Input: part model. Units: mm. Frame: model coordinates. Face numbers are marked on the shaded views. A direction names the side the tool comes from. Coordinates: 2 decimals unless noted, no trailing zeros. Order: outer loops, then holes, each group sorted by start corner. A loop starts at its lowest first (then second) coordinate and runs counter-clockwise, first axis right, second up. Notation, with made-up numbers: (57, -10) -> (69, -10) arc R27 ccw to (69, 20) -> close; hole circle Ø7 at (41.25, 23.25). An arc over 180 degrees is marked (long way). Answer as CSV lines item,"result".
from build123d import *

# Parameters (mm, degrees)
SALIENTE_EXTRUIR1_DEPTH = 30
SALIENTE_EXTRUIR2_DEPTH = 90
CORTAR_EXTRUIR1_DEPTH   = 138.564065
MATRIZC1_COUNT          = 6
CROQUIS4_R              = 15.75
CORTAR_EXTRUIR2_DEPTH   = 103.923048
MATRIZC2_COUNT          = 6


with BuildPart() as part:
    # Croquis1 → Saliente-Extruir1 (new body)
    with BuildSketch(Plane(origin=(0, 0, 0), x_dir=(1, 0, 0), z_dir=(0, 1, 0))):
        Polygon((40, 69.282032303), (-40, 69.282032303), (-80, 0), (-40, -69.282032303), (40, -69.282032303), (80, 0), align=None)
    extrude(amount=SALIENTE_EXTRUIR1_DEPTH)

    # Croquis2 → Saliente-Extruir2 (add)
    with BuildSketch(Plane(origin=(0, 0, 0), x_dir=(1, 0, 0), z_dir=(0, 1, 0))):
        Polygon((20, 34.641016151), (-20, 34.641016151), (-40, 0), (-20, -34.641016151), (20, -34.641016151), (40, 0), align=None)
    extrude(amount=SALIENTE_EXTRUIR2_DEPTH)

    # Croquis3 → Cortar-Extruir1 (cut)
    with BuildSketch(Plane(origin=(60, 0, 34.641016151), x_dir=(0.5, 0, -0.866025404), z_dir=(0.866025404, 0, 0.5))):
        with BuildLine():
            Line((-10, 25), (10, 25))
            ThreePointArc((10, 25), (20, 15), (10, 5))
            Line((10, 5), (-10, 5))
            ThreePointArc((-10, 5), (-20, 15), (-10, 25))
        make_face()
    cortar_extruir1 = extrude(amount=-CORTAR_EXTRUIR1_DEPTH, mode=Mode.SUBTRACT)

    # MatrizC1: Cortar-Extruir1 ×6 about axis
    matrizc1_axis = Axis((0, 0, 0), (0, 1, 0))
    for i in range(1, MATRIZC1_COUNT):
        add(cortar_extruir1.rotate(matrizc1_axis, i * 360 / MATRIZC1_COUNT), mode=Mode.SUBTRACT)

    # Croquis4 → Cortar-Extruir2 (cut)
    with BuildSketch(Plane(origin=(30, 0, -17.320508076), x_dir=(-0.5, 0, -0.866025404), z_dir=(0.866025404, 0, -0.5))):
        with Locations((0, 60)):
            Circle(CROQUIS4_R)
    cortar_extruir2 = extrude(amount=-CORTAR_EXTRUIR2_DEPTH, mode=Mode.SUBTRACT)

    # MatrizC2: Cortar-Extruir2 ×6 about axis
    matrizc2_axis = Axis((0, 90, 0), (0, 1, 0))
    for i in range(1, MATRIZC2_COUNT):
        add(cortar_extruir2.rotate(matrizc2_axis, i * 360 / MATRIZC2_COUNT), mode=Mode.SUBTRACT)


solid = part.part
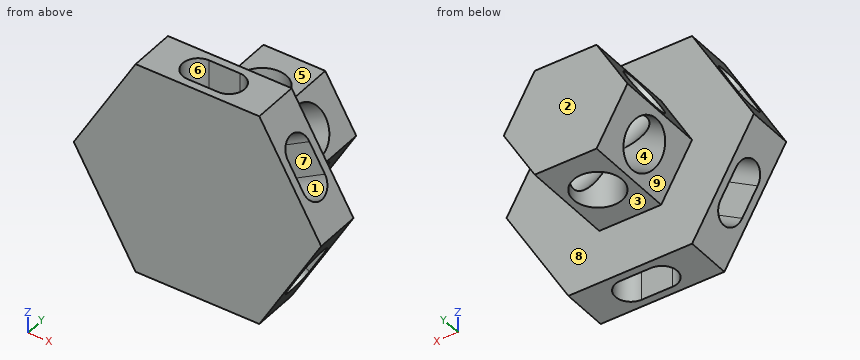
1. Mould query, pull axis Z, two halves, no side actions, for the marked faces 1, 2, 3 and 4. Classes: released by +Z, released by -Z, zero draft, split by the parting line, or undercut.
Findings:
face 1,"undercut"
face 2,"zero draft"
face 3,"released by -Z"
face 4,"undercut"
2. Cut plane B-B (z = -60). Return the cut outline in (x, y).
Findings:
outline,"(-45.36, 0) -> (45.36, 0) -> (45.36, 30) -> (-45.36, 30) -> close; hole (-10, 5) -> (10, 5) arc R10 ccw to (10, 25) -> (-10, 25) arc R10 ccw to start"
3. Cut plane C-C (y = 83). Return the cut outline in (x, z).
Findings:
outline,"(-40, 0) -> (-20, -34.64) -> (20, -34.64) -> (40, 0) -> (20, 34.64) -> (-20, 34.64) -> close"
4. Cut plane D-D (x = 42). State how many separate pieces and enclosed holes the cut face has, plus the area to 3 significant figures.
Findings:
separate pieces,"1"
enclosed holes,"2"
area,"2,300 mm2"
5. Contact query for flat-ended pins moving along their axis: pin 1 (1 mm diameter, centred on y = 13.5, z = -53.5, fed in from +X); pin 2 (1 mm diameter, centred on x = 14, y = 37.5, fed in from -Z); pin 3 (6 mm diameter, centred on x = -29, y = 34, fed in from -Z). Output: stop coordinate, or through.
Findings:
pin 1,"stops at x = 49.4"
pin 2,"stops at z = -34.64"
pin 3,"stops at z = -24.25"
6. Ray query, line 1 along Y through (x, z) = (0, 24); line 2 along Y through (x, z) = (-24, 19); line 3 along Y through (x, z) = (8.5, 38.5). Return the intervals inside material, ascending.
Findings:
line 1,"y = 0 to 5, 25 to 44.25, 75.75 to 90"
line 2,"y = 0 to 5, 25 to 44.89, 75.11 to 90"
line 3,"y = 0 to 5, 25 to 30"
7. Reachability of the marked faces 5, 6, 7, 8 and 9 from +Z, -Z, +X, -X, +Y, -Y: full face, straight path, thin tool, end or side. Return the list, or none.
Findings:
face 5,"+Z, +X, -X, +Y"
face 6,"+Z, -Z"
face 7,"none"
face 8,"+Y"
face 9,"-Z, -X, +Y"
8. Cut plane A-A (y = 60). Return the cut outline in (x, z) (3 decimals).
Findings:
outline,"(-40, 0) -> (-37.875, -3.681) -> (-31.5, 0) -> (-37.875, 3.681) -> close; (-22.125, -30.96) -> (-20, -34.641) -> (-15.75, -34.641) -> (-15.75, -27.28) -> close; (-22.125, 30.96) -> (-15.75, 27.28) -> (-15.75, 34.641) -> (-20, 34.641) -> close; (15.75, -34.641) -> (20, -34.641) -> (22.125, -30.96) -> (15.75, -27.28) -> close; (15.75, 27.28) -> (22.125, 30.96) -> (20, 34.641) -> (15.75, 34.641) -> close; (31.5, 0) -> (37.875, -3.681) -> (40, 0) -> (37.875, 3.681) -> close"
